from build123d import *

# Parameters (mm, degrees)
SKETCH_1_R      = 85.5
SKETCH_1_R_2    = 72.5
SKETCH_1_R_3    = 2.65
EXTRUDE_2_DEPTH = 10
SKETCH_2_R      = 101
SKETCH_2_R_2    = 85.5
SKETCH_2_R_3    = 2.65
EXTRUDE_3_DEPTH = 10


with BuildPart() as part:
    # 草图1 → 凸台-拉伸2 (new body)
    with BuildSketch(Plane(origin=(0, 0, 0), x_dir=(1, 0, 0), z_dir=(0, 1, 0))):
        with Locations(Location((0, 0, 0), (0, 0, 270))):
            Circle(SKETCH_1_R)
        with Locations(Location((0, 0, 0), (0, 0, 270))):
            Circle(SKETCH_1_R_2, mode=Mode.SUBTRACT)
        with Locations(Location((0, 79, 0), (0, 0, 270))):
            Circle(SKETCH_1_R_3, mode=Mode.SUBTRACT)
        with Locations(Location((79, 0, 0), (0, 0, 270))):
            Circle(SKETCH_1_R_3, mode=Mode.SUBTRACT)
        with Locations(Location((0, -79, 0), (0, 0, 270))):
            Circle(SKETCH_1_R_3, mode=Mode.SUBTRACT)
        with Locations(Location((-79, 0, 0), (0, 0, 270))):
            Circle(SKETCH_1_R_3, mode=Mode.SUBTRACT)
    extrude(amount=EXTRUDE_2_DEPTH)

    # 草图2 → 凸台-拉伸3 (add)
    with BuildSketch(Plane(origin=(0, -2, 0), x_dir=(-1, 0, 0), z_dir=(0, -1, 0))):
        with Locations(Location((0, 0, 0), (0, 0, 90))):
            Circle(SKETCH_2_R)
        with Locations(Location((0, 0, 0), (0, 0, 90))):
            Circle(SKETCH_2_R_2, mode=Mode.SUBTRACT)
        with Locations(Location((0, 93.25, 0), (0, 0, 90))):
            Circle(SKETCH_2_R_3, mode=Mode.SUBTRACT)
        with Locations(Location((93.25, 0, 0), (0, 0, 90))):
            Circle(SKETCH_2_R_3, mode=Mode.SUBTRACT)
        with Locations(Location((0, -93.25, 0), (0, 0, 90))):
            Circle(SKETCH_2_R_3, mode=Mode.SUBTRACT)
        with Locations(Location((-93.25, 0, 0), (0, 0, 90))):
            Circle(SKETCH_2_R_3, mode=Mode.SUBTRACT)
    extrude(amount=-EXTRUDE_3_DEPTH)


solid = part.part
Part model, mm, in its own coordinate system. A direction names the side the tool comes from. Coordinates: 2 decimals unless noted, no trailing zeros. Write each loop counter-clockwise with the first axis right and the second up, starting at its lowest first coordinate (ties: lowest second). Pieces come first, ordered by that corner, then holes. Notation, with made-up numbers: M 58,30.25 L 76,30.25 A31 cw 76,60.25 Z; hole C -2.75,-37.75 d8. An arc over 180 degrees is marked long. Return JSON: item names as keys, results as strings.
1. Saw through at A-A, the plane z = 0. Count the separate pieces of the cut face and the enclosed holes in it, then the cut area to 3 significant figures.
Determined:
{"separate pieces": "6", "enclosed holes": "0", "area": "358 mm²"}
2. Pull direction Z, two halves, no side cores. Call faces 4 (the face through (-95.84, 2.93, 0.57)), 5 (the face through (84.772, 8.986, -11.13)), 6 (the face through (23, -2, 83)): pulls with the +Z half, pulls with the -Z half, needs draft (parallel to the pull), parting line crosses it, or undercut.
Determined:
{"face 4": "undercut", "face 5": "parting line crosses it", "face 6": "needs draft"}
3. Flat gauge pins, fed straight in: pin 1 Ø2 at (y, z) = (8, -75) entering from +X; pin 2 Ø4 at (x, z) = (-93.25, 0) entering from +Y; pin 3 Ø8.5 at (x, z) = (0, -93.25) entering from +Y; pin 4 Ø5 at (x, y) = (29.5, 1) entering from +Z. Where does each tip first touch, or does it go through?
Determined:
{"pin 1": "x = 68.74", "pin 2": "through", "pin 3": "y = 8", "pin 4": "z = 97.32"}
4. Saw through at C-C, the plane z = -93.25. Write the cut outline in (x, y).
Determined:
{"outline": "M -38.8,-2 L -2.65,-2 L -2.65,8 L -38.8,8 Z; M 2.65,-2 L 38.8,-2 L 38.8,8 L 2.65,8 Z"}
5. 3-axis set-ups, long thin cutter, end or side, ignore diameter. For faces 1 (the face through (23, 8, 83)), 2 (the face through (84.772, -1.014, 11.13)), 3 (the face through (76.41, 4.93, -0.57)): which of +Z, -Z, +X, -X, +Y, -Y reach the whole face in a straight line?
Determined:
{"face 1": "+Y", "face 2": "-Y", "face 3": "+Y, -Y"}
6. Saw through at D-D, the plane x = -93.25. Write the cut outline in (y, z).
Determined:
{"outline": "M -2,-38.8 L 8,-38.8 L 8,-2.65 L -2,-2.65 Z; M -2,2.65 L 8,2.65 L 8,38.8 L -2,38.8 Z"}
7. Saw through at B-B, the plane x = -15. Write the cut outline in (y, z), then the cut area to 3 significant figures.
Determined:
{"outline": "M -2,-99.88 L 8,-99.88 L 8,-84.17 L 10,-84.17 L 10,-70.93 L 0,-70.93 L 0,-84.17 L -2,-84.17 Z; M -2,84.17 L 0,84.17 L 0,70.93 L 10,70.93 L 10,84.17 L 8,84.17 L 8,99.88 L -2,99.88 Z", "area": "579 mm²"}
8. Probe L1, parallel to X at y = 4.75, z = 0; L2, parallel to Y at x = 8, z = 75; L3, parallel to X at y = 1, z = 56. List the from-to ranges inside material, lowest first.
Determined:
{"L1": "-101 to -95.9, -90.6 to -81.65, -76.35 to -72.5, 72.5 to 76.35, 81.65 to 90.6, 95.9 to 101", "L2": "0 to 10", "L3": "-84.05 to -46.05, 46.05 to 84.05"}
